from build123d import *

# Parameters (mm, degrees)
BOSS_EXTRUDE1_DEPTH = 3.175
SKETCH2_W           = 50.8
SKETCH2_H           = 25.4
BOSS_EXTRUDE2_DEPTH = 6.35


with BuildPart() as part:
    # Sketch1 → Boss-Extrude1 (new, symmetric)
    with BuildSketch(Plane.XY):
        with BuildLine():
            Line((12.7, 25.4), (25.4, 25.4))
            Line((25.4, 25.4), (25.4, -25.4))
            Line((25.4, -25.4), (-25.4, -25.4))
            Line((-25.4, -25.4), (-25.4, 25.4))
            Line((-25.4, 25.4), (-12.7, 25.4))
            ThreePointArc((-12.7, 25.4), (0, 12.7), (12.7, 25.4))
        make_face()
    extrude(amount=BOSS_EXTRUDE1_DEPTH, both=True)

    # Sketch2 → Boss-Extrude2 (add)
    with BuildSketch(Plane.XY.offset(3.175)):
        with Locations((0, -12.7)):
            Rectangle(SKETCH2_W, SKETCH2_H)
    extrude(amount=BOSS_EXTRUDE2_DEPTH)


solid = part.part
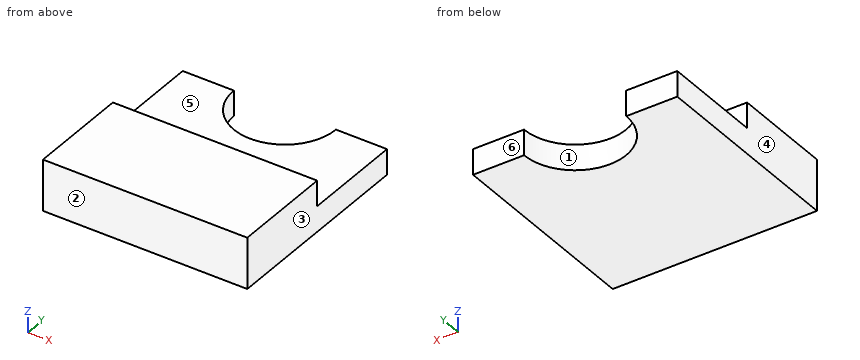
Geometry check sheet. Reference: the model listing, model coordinates, mm. Face numbers are marked on the shaded views. A direction names the side the tool comes from. Coordinates: 2 decimals unless noted, no trailing zeros. Order: outer loops, then holes, each group sorted by start corner. A loop starts at its lowest first (then second) coordinate and runs counter-clockwise, first axis right, second up. Notation, with made-up numbers: (46, 27) - (64, 27) arc R25 cw to (64, 43) - close; hole circle Ø2 at (64.5, 3). An arc over 180 degrees is marked (long way). Answer in a Markdown table with one row per item. Add a question column.
1) Material ranges on line 1 along Y through (x, z) = (-13, 5); line 2 along Z through (x, y) = (6.5, 13.5) (3 decimals); line 3 along X through (y, z) = (21, -2.5), recorded low to high. Write a range as [from, to].
2) Cross-section at C-C, the plane z = 2. Record the cut outline in (x, y).
3) Cross-section at A-A, the plane y = 22.5. Record the cut outline in (x, z) (3 decimals).
4) Cross-section at B-B, the plane x = 0. Record the cut outline in (y, z) (3 decimals).
5) Gauge pin test, flat ends, axial feed: P1, Ø3, axis at x = 6.5, z = 6.5, coming from the +Y side; P2, Ø12.5, axis at x = -3, y = 17, coming from the +Z side (3 decimals). Record the tip position at first contact, or that the pin passes through.
6) Set-up check for the marked faces 5 and 6: record each of +Z, -Z, +X, -X, +Y, -Y from which the full face is reachable in a straight line by a thin tool's end or side.
7) Release check for a two-part mould opening along X. For the marked faces 1, 2, 3 and 4 record: +X half, -X half, draft (parallel to the pull), parting line (faces both ways), or undercut.
Check result:
| question | item | result |
|---|---|---|
| 1 | line 1 | y = [-25.4, 0] |
| 1 | line 2 | z = [-3.175, 3.175] |
| 1 | line 3 | x = [-25.4, -11.91], [11.91, 25.4] |
| 2 | outline | (-25.4, -25.4) - (25.4, -25.4) - (25.4, 25.4) - (12.7, 25.4) arc R12.7 cw to (-12.7, 25.4) - (-25.4, 25.4) - close |
| 3 | outline | (-25.4, -3.175) - (-12.364, -3.175) - (-12.364, 3.175) - (-25.4, 3.175) - close; (12.364, -3.175) - (25.4, -3.175) - (25.4, 3.175) - (12.364, 3.175) - close |
| 4 | outline | (-25.4, -3.175) - (12.7, -3.175) - (12.7, 3.175) - (0, 3.175) - (0, 9.525) - (-25.4, 9.525) - close |
| 5 | P1 | stops at y = 0 |
| 5 | P2 | stops at z = 3.175 |
| 6 | face 5 | +Z, +X, -X, +Y |
| 6 | face 6 | +Z, -Z, +X, -X, +Y |
| 7 | face 1 | undercut |
| 7 | face 2 | draft |
| 7 | face 3 | +X half |
| 7 | face 4 | -X half |
